Read the model definition and answer for the solid it produces. Units are mm, in the model's axes. A direction names the side the tool comes from. Give positions to 0.01 mm unless a question says otherwise; leave off trailing zeros. Loops run counter-clockwise (first coordinate to the right, second up) from the corner with the lowest first, then second, coordinate; pieces in that order, holes last. Notation, with made-up numbers: (-2, -19.75) - (47, -19.75) arc R16 ccw to (47, -5.75) - close; hole circle Ø1 at (80.25, -7). An arc over 180 degrees is marked (long way). Write item = value, one per line.
```python
from build123d import *

# Parameters (mm, degrees)
BOSS_EXTRUDE1_DEPTH = 25.4
SKETCH2_R           = 1.8288
CUT_EXTRUDE1_DEPTH  = 12.7
SKETCH3_R           = 1.8288
CUT_EXTRUDE2_DEPTH  = 12.7


with BuildPart() as part:
    # Sketch1 → Boss-Extrude1 (new body)
    with BuildSketch(Plane(origin=(0, 0, 0), x_dir=(0, 0, -1), z_dir=(1, 0, 0))):
        Polygon((0, 6.096), (0, 0), (6.35, 0), (6.35, 2.921), (12.7, 2.921), (12.7, 0), (19.05, 0), (19.05, -6.604), (34.925, -6.604), (34.925, 6.096), align=None)
    extrude(amount=BOSS_EXTRUDE1_DEPTH)

    # Sketch2 → Cut-Extrude1 (cut)
    with BuildSketch(Plane(origin=(0, 0, -34.925), x_dir=(-1, 0, 0), z_dir=(0, 0, -1))):
        with Locations((-19.05, 2.921)):
            Circle(SKETCH2_R)
        with Locations((-6.35, 2.921)):
            Circle(SKETCH2_R)
        with Locations((-19.05, -3.429)):
            Circle(SKETCH2_R)
        with Locations((-6.35, -3.429)):
            Circle(SKETCH2_R)
    extrude(amount=-CUT_EXTRUDE1_DEPTH, mode=Mode.SUBTRACT)

    # Sketch3 → Cut-Extrude2 (cut)
    with BuildSketch(Plane.XZ):
        with Locations((3.175, -3.175)):
            Circle(SKETCH3_R)
        with Locations((3.175, -15.875)):
            Circle(SKETCH3_R)
        with Locations((22.225, -3.175)):
            Circle(SKETCH3_R)
        with Locations((22.225, -15.875)):
            Circle(SKETCH3_R)
    extrude(amount=-CUT_EXTRUDE2_DEPTH, mode=Mode.SUBTRACT)


solid = part.part
```
1) A cutting plane is placed at D-D on x = 23.25. Determine the outline of the cut face in (y, z) (3 decimals).
Output:
outline = (-6.604, -34.925) - (6.096, -34.925) - (6.096, -17.39) - (0, -17.39) - (0, -19.05) - (-6.604, -19.05) - close; (0, -14.36) - (6.096, -14.36) - (6.096, -4.69) - (0, -4.69) - (0, -6.35) - (2.921, -6.35) - (2.921, -12.7) - (0, -12.7) - close; (0, -1.66) - (6.096, -1.66) - (6.096, 0) - (0, 0) - close
2) A cutting plane is placed at C-C on y = 0.5. Determine the outline of the cut face in (x, z) (3 decimals), then the cut area to 3 significant figures.
Output:
outline = (0, -34.925) - (25.4, -34.925) - (25.4, -12.7) - (0, -12.7) - close; (0, -6.35) - (25.4, -6.35) - (25.4, 0) - (0, 0) - close; hole circle Ø3.658 at (3.175, -15.875); hole circle Ø3.658 at (3.175, -3.175); hole circle Ø3.658 at (22.225, -15.875); hole circle Ø3.658 at (22.225, -3.175)
area = 684 mm²
3) A cutting plane is placed at A-A on y = 4. Determine the outline of the cut face in (x, z) (3 decimals), then the cut area to 3 significant figures.
Output:
outline = (0, -34.925) - (4.873, -34.925) - (4.873, -22.225) - (7.827, -22.225) - (7.827, -34.925) - (17.573, -34.925) - (17.573, -22.225) - (20.527, -22.225) - (20.527, -34.925) - (25.4, -34.925) - (25.4, 0) - (0, 0) - close; hole circle Ø3.658 at (3.175, -15.875); hole circle Ø3.658 at (3.175, -3.175); hole circle Ø3.658 at (22.225, -15.875); hole circle Ø3.658 at (22.225, -3.175)
area = 770 mm²
4) A tool of negligible diameter and unlimited length cuts with its end or side. For faces 4 (the face through (6, 3, -22.225)), 5 (the face through (13, 2.921, -9)), 6 (the face through (13, 0, -3)), from which of +Z, -Z, +X, -X, +Y, -Y can it reach the whole face along a straight path? Write none if from no direction.
Output:
face_4 = -Z
face_5 = +X, -X, -Y
face_6 = +Z, +X, -X, -Y
5) A cutting plane is placed at B-B on x = 19.05. Determine the outline of the cut face in (y, z) (3 decimals), then the cut area to 3 significant figures.
Output:
outline = (-6.604, -34.925) - (-5.258, -34.925) - (-5.258, -22.225) - (-1.6, -22.225) - (-1.6, -34.925) - (1.092, -34.925) - (1.092, -22.225) - (4.75, -22.225) - (4.75, -34.925) - (6.096, -34.925) - (6.096, 0) - (0, 0) - (0, -6.35) - (2.921, -6.35) - (2.921, -12.7) - (0, -12.7) - (0, -19.05) - (-6.604, -19.05) - close
area = 206 mm²
6) Find the intervals of material crossed by probe 1 along Y at (x, z) = (19.05, -32); probe 2 along Z at (x, y) = (19.5, 2.5) (3 decimals); probe 3 along Z at (x, y) = (16, 1.75) (3 decimals), in increasing order.
Output:
probe_1 = -6.6 to -5.26, -1.6 to 1.09, 4.75 to 6.1
probe_2 = -22.225 to -12.7, -6.35 to 0
probe_3 = -34.925 to -12.7, -6.35 to 0
7) Each of these flat-tipped pins is pushed along its axis until it touches: P1, Ø1.8, axis at x = 19.5, y = 3.5, coming from the -Z side (3 decimals); P2, Ø1, axis at x = 22.5, z = -7, coming from the -Y side; P3, Ø3, axis at x = 14.5, z = -15.5, coming from the -Y side. Where does it stop, or does it pass through?
Output:
P1 = -22.225
P2 = 2.92
P3 = 0
8) The mould has two halves that part along X. Classify faces 1 (the face through (25.4, 1, -21)), 2 (the face through (13, 6.096, -18)), 3 (the face through (21.83, 3.01, -17.66)): pulls with the +X half, pulls with the -X half, needs draft (parallel to the pull), parting line crosses it, or undercut.
Output:
face_1 = pulls with the +X half
face_2 = needs draft
face_3 = undercut
